Input: part model. Units: mm. Frame: model coordinates. A direction names the side the tool comes from. Round coordinates to 2 decimals unless told otherwise and drop trailing zeros. Loops run counter-clockwise (first coordinate to the right, second up) from the corner with the lowest first, then second, coordinate; pieces in that order, holes last.
1) Access query for faces 5 (the face through (-18, -21, 35.4)), 6 (the face through (-8.618, -107.849, -20.784)), 7 (the face through (-20.5, -52, 33.7)). Directions: +Z, -Z, +X, -X, +Y, -Y. A direction counts if a zero-diameter tool reaches every point of the face in a straight line with its end or side. Return the directions, or none.
2) Ray query, line 1 along Y through (x, z) = (-22, -19); line 2 along Y through (x, z) = (13, 5); line 3 along Z through (x, y) = (-1, -76.5). Return the intervals inside material, ascending.
3) Draft query along Y for faces 1 (the face through (0, 21, 20)), 2 (the face through (-28, -41, 31)), 3 (the face through (-39.5, -52, -0.5)), 4 (the face through (12, 25, 0)). Return one class per face: pulls with the +Y half, pulls with the -Y half, needs draft (parallel to the pull), parting line crosses it, or undercut.
4) First-contact query: pin 1 (10 mm diameter, centred on x = -12, y = 33.5, fed in from +Z); pin 2 (1.5 mm diameter, centred on y = 30.5, z = 16.5, fed in from -X); pin 3 (4 mm diameter, centred on y = 4, z = -21, fed in from +X); pin 4 (10 mm diameter, centred on x = -26.5, y = -63, fed in from +Z). Flat tips, straight axial feed; report the tip coordinate or a pass-through.
5) Section A-A, the plane y = 11. Return loops of the section in (x, z).
from build123d import *

# Parameters (mm, degrees)
SKETCH2_R            = 39.5
BOSS_EXTRUDE1_DEPTH  = 1
SKETCH4_R            = 41.25
BOSS_EXTRUDE2_DEPTH  = 1
SKETCH5_R            = 42
BOSS_EXTRUDE3_DEPTH  = 7
SKETCH6_R            = 35
BOSS_EXTRUDE4_DEPTH  = 7
BOSS_EXTRUDE7_DEPTH  = 3
CIRPATTERN2_COUNT    = 12
SKETCH8_R            = 15
BOSS_EXTRUDE8_DEPTH  = 50
SKETCH9_W            = 24
SKETCH9_H            = 40
BOSS_EXTRUDE9_DEPTH  = 42
BOSS_EXTRUDE10_START = -24
BOSS_EXTRUDE10_DEPTH = 24
SKETCH11_R           = 15
BOSS_EXTRUDE11_DEPTH = 15.5
BOSS_EXTRUDE12_START = 15.5
SKETCH12_R           = 15
BOSS_EXTRUDE12_DEPTH = 15.5
SKETCH13_R           = 22.5
BOSS_EXTRUDE13_DEPTH = 3.75


with BuildPart() as part:
    # Sketch1 → Revolve1 (revolve)
    with BuildSketch(Plane.XY):
        with BuildLine():
            Line((0, 0), (-35, 0))
            ThreePointArc((-35, 0), (-39.657515479, -9.46062113), (-40, -20))
            Line((-40, -20), (0, -20))
            Line((0, -20), (0, 0))
        make_face()
    revolve(axis=Axis((0, 0, 0), (0, -1, 0)))

    # Sketch2 → Boss-Extrude1 (add)
    with BuildSketch(Plane.XZ.offset(20)):
        Circle(SKETCH2_R)
    extrude(amount=BOSS_EXTRUDE1_DEPTH)

    # Sketch3 → Revolve2 (revolve)
    with BuildSketch(Plane(origin=(0, 0, 0), x_dir=(0, 0, -1), z_dir=(1, 0, 0)), mode=Mode.PRIVATE) as revolve2_sk:
        with BuildLine():
            Line((0, -21), (-40, -21))
            ThreePointArc((-40, -21), (-42.384109041, -30.861589096), (-42, -41))
            Line((-42, -41), (0, -41))
            Line((0, -41), (0, -21))
        make_face()
    revolve(revolve2_sk.sketch.rotate(Axis((0, -21, 0), (0, -1, 0)), 90), axis=Axis((0, -21, 0), (0, -1, 0)))

    # Sketch4 → Boss-Extrude2 (add)
    with BuildSketch(Plane.XZ.offset(41)):
        with Locations(Location((0, 0, 0), (0, 0, 270))):
            Circle(SKETCH4_R)
    extrude(amount=BOSS_EXTRUDE2_DEPTH)

    # Sketch5 → Boss-Extrude3 (add)
    with BuildSketch(Plane.XZ.offset(42)):
        with Locations(Location((0, 0, 0), (0, 0, 270))):
            Circle(SKETCH5_R)
    extrude(amount=BOSS_EXTRUDE3_DEPTH)

    # Sketch6 → Boss-Extrude4 (add)
    with BuildSketch(Plane.XZ.offset(49)):
        with Locations(Location((0, 0, 0), (0, 0, 270))):
            Circle(SKETCH6_R)
    extrude(amount=BOSS_EXTRUDE4_DEPTH)

    # Sketch7 → Boss-Extrude7 (add)
    with BuildSketch(Plane.XZ.offset(49)):
        Polygon((40.75, 0), (39.625, 1.948557159), (37.375, 1.948557159), (36.25, 0), (37.375, -1.948557159), (39.625, -1.948557159), align=None)
        Polygon((39.047649731, 0.948557159), (37.952350269, 0.948557159), (37.404700538, 0), (37.952350269, -0.948557159), (39.047649731, -0.948557159), (39.595299462, 0), align=None, mode=Mode.SUBTRACT)
    boss_extrude7 = extrude(amount=BOSS_EXTRUDE7_DEPTH)

    # CirPattern2: Boss-Extrude7 ×12 about axis
    cirpattern2_axis = Axis((0, 0, 0), (0, 1, 0))
    for i in range(1, CIRPATTERN2_COUNT):
        add(boss_extrude7.rotate(cirpattern2_axis, i * 360 / CIRPATTERN2_COUNT))

    # Sketch8 → Boss-Extrude8 (add)
    with BuildSketch(Plane.XZ.offset(56)):
        with Locations(Location((0, 0, 0), (0, 0, 270))):
            Circle(SKETCH8_R)
    extrude(amount=BOSS_EXTRUDE8_DEPTH)

    # Sketch9 → Boss-Extrude9 (add)
    with BuildSketch(Plane(origin=(0, 0, 0), x_dir=(1, 0, 0), z_dir=(0, 1, 0))):
        Rectangle(SKETCH9_W, SKETCH9_H)
    extrude(amount=BOSS_EXTRUDE9_DEPTH)

    # Sketch10 → Boss-Extrude10 (add)
    with BuildSketch(Plane.ZY.offset(12).offset(BOSS_EXTRUDE10_START)):
        with BuildLine():
            Line((-20, 42), (20, 42))
            ThreePointArc((20, 42), (0, 62), (-20, 42))
        make_face()
    extrude(amount=BOSS_EXTRUDE10_DEPTH)

    # Sketch11 → Boss-Extrude11 (add)
    with BuildSketch(Plane.ZY.offset(12)):
        with Locations(Location((0, 42, 0), (0, 0, 90))):
            Circle(SKETCH11_R)
    extrude(amount=BOSS_EXTRUDE11_DEPTH)

    # Sketch12 → Boss-Extrude12 (add)
    with BuildSketch(Plane(origin=(12, 0, 0), x_dir=(0, 0, -1), z_dir=(1, 0, 0)).offset(BOSS_EXTRUDE12_START)):
        with Locations(Location((0, 42, 0), (0, 0, 90))):
            Circle(SKETCH12_R)
    extrude(amount=-BOSS_EXTRUDE12_DEPTH)

    # Sketch13 → Boss-Extrude13 (add)
    with BuildSketch(Plane.XZ.offset(106)):
        with Locations(Location((0, 0, 0), (0, 0, 270))):
            Circle(SKETCH13_R)
    extrude(amount=BOSS_EXTRUDE13_DEPTH)


solid = part.part
Final values:
1. face 5: none
1. face 6: -Y
1. face 7: +Z, -X, -Y
2. line 1: y = -56 to 0
2. line 2: y = -109.75 to 0, 27.86 to 56.14
2. line 3: z = -14.97 to 14.97
3. face 1: needs draft
3. face 2: undercut
3. face 3: pulls with the -Y half
3. face 4: undercut
4. pin 1: stops at z = 20
4. pin 2: stops at x = -12
4. pin 3: stops at x = 12
4. pin 4: passes through
5. outline: (-12, -20) - (12, -20) - (12, 20) - (-12, 20) - close
